Input: part model. Units: mm. Frame: model coordinates. A direction names the side the tool comes from. Coordinates: 2 decimals unless noted, no trailing zeros. Write each loop counter-clockwise with the first axis right and the second up, starting at its lowest first coordinate (ties: lowest second). Pieces come first, ordered by that corner, then holes. Notation, with made-up numbers: M 22.25,52 L 55.25,52 A37 cw 55.25,90 Z; hole C 69,25 d11. An arc over 180 degrees is marked long. Use one line per item in the form item = value.
from build123d import *

# Parameters (mm, degrees)
SKETCH_1_W                  = 78
SKETCH_1_H                  = 119.63
SKETCH_1_R                  = 22.5
EXTRUDE_1_DEPTH             = 8
HOLE_WIZARD_M5_1_AT_2_COUNT = 2
HOLE_WIZARD_M5_1_AT_2_PITCH = 58
SKETCH_4_W                  = 78
SKETCH_4_H                  = 23.52391086
EXTRUDE_2_DEPTH             = 8
SKETCH_5_W                  = 78
SKETCH_5_H                  = 8.43
EXTRUDE_3_DEPTH             = 10
SKETCH_6_W                  = 78
SKETCH_6_H                  = 18
CUT_EXTRUDE_1_DEPTH         = 0.43
SKETCH_7_R                  = 2.75
CUT_EXTRUDE_2_DEPTH         = 9
HOLE_WIZARD_M5_2_AT_2_COUNT = 2
HOLE_WIZARD_M5_2_AT_2_PITCH = 90


with BuildPart() as part:
    # 草图1 → 凸台-拉伸1 (new body)
    with BuildSketch(Plane.XY):
        with Locations((-39, 59.815)):
            Rectangle(SKETCH_1_W, SKETCH_1_H)
        with Locations((-39, 59.815)):
            Circle(SKETCH_1_R, mode=Mode.SUBTRACT)
    extrude(amount=EXTRUDE_1_DEPTH)

    # 草图3 → M5 螺纹孔1 (revolve, cut)
    with BuildSketch(Plane(origin=(-68, 119.63, 4), x_dir=(0, 0, 1), z_dir=(1, 0, 0))):
        Polygon((0, 0), (0, 13.6618073), (2.1, 12.4), (2.1, 0), align=None)
    hole_wizard_m5_1 = revolve(axis=Axis((-68, 125.98, 4), (0, -1, 0)), mode=Mode.SUBTRACT)

    # M5 螺纹孔1 at 2: M5 螺纹孔1 ×2
    with Locations(*[(i * HOLE_WIZARD_M5_1_AT_2_PITCH, 0, 0) for i in range(1, HOLE_WIZARD_M5_1_AT_2_COUNT)]):
        add(hole_wizard_m5_1, mode=Mode.SUBTRACT)

    # 镜向1: M5 螺纹孔1 across plane
    add(hole_wizard_m5_1.mirror(Plane.ZX.offset(59.815)), mode=Mode.SUBTRACT)

    # 镜向1 copy 1 sketch → 镜向1 copy 1 (revolve, cut)
    with BuildSketch(Plane(origin=(-10, 0, 4), x_dir=(0, 0, 1), z_dir=(1, 0, 0))):
        Polygon((0, 0), (0, -13.6618073), (2.1, -12.4), (2.1, 0), align=None)
    revolve(axis=Axis((-10, -6.35, 4), (0, -1, 0)), mode=Mode.SUBTRACT)

    # 草图4 → 凸台-拉伸2 (add)
    with BuildSketch(Plane.XY.offset(8)):
        with Locations((-39, 107.86804457)):
            Rectangle(SKETCH_4_W, SKETCH_4_H)
    extrude(amount=-EXTRUDE_2_DEPTH)

    # 草图5 → 凸台-拉伸3 (add)
    with BuildSketch(Plane(origin=(0, 0, 0), x_dir=(-1, 0, 0), z_dir=(0, 0, -1))):
        with Locations((39, 115.415)):
            Rectangle(SKETCH_5_W, SKETCH_5_H)
    extrude(amount=EXTRUDE_3_DEPTH)

    # 草图6 → 切除-拉伸1 (cut)
    with BuildSketch(Plane(origin=(0, 119.63, 0), x_dir=(1, 0, 0), z_dir=(0, 1, 0))):
        with Locations((-39, 1)):
            Rectangle(SKETCH_6_W, SKETCH_6_H)
    extrude(amount=-CUT_EXTRUDE_1_DEPTH, mode=Mode.SUBTRACT)

    # 草图7 → 切除-拉伸2 (cut, through all)
    with BuildSketch(Plane.XZ.offset(-111.2)):
        with Locations((-59, -5)):
            Circle(SKETCH_7_R)
        with Locations((-19, -5)):
            Circle(SKETCH_7_R)
    extrude(amount=-CUT_EXTRUDE_2_DEPTH, mode=Mode.SUBTRACT)

    # 草图9 → M5 螺纹孔2 (revolve, cut)
    with BuildSketch(Plane(origin=(-78, 7, 4), x_dir=(0, 0, 1), z_dir=(0, 1, 0))):
        Polygon((0, 0), (0, 7.2618073), (2.1, 6), (2.1, 0), align=None)
    hole_wizard_m5_2 = revolve(axis=Axis((-84.35, 7, 4), (1, 0, 0)), mode=Mode.SUBTRACT)

    # M5 螺纹孔2 at 2: M5 螺纹孔2 ×2
    with Locations(*[(0, 0, -i * HOLE_WIZARD_M5_2_AT_2_PITCH) for i in range(1, HOLE_WIZARD_M5_2_AT_2_COUNT)]):
        add(hole_wizard_m5_2, mode=Mode.SUBTRACT)

    # 镜向2: M5 螺纹孔2 across plane
    add(hole_wizard_m5_2.mirror(Plane(origin=(-39, 0, 0), x_dir=(0, 0, 1), z_dir=(1, 0, 0))), mode=Mode.SUBTRACT)

    # 镜向2 copy 1 sketch → 镜向2 copy 1 (revolve, cut)
    with BuildSketch(Plane(origin=(0, 7, -86), x_dir=(0, 0, 1), z_dir=(0, 1, 0))):
        Polygon((0, 0), (0, -7.2618073), (2.1, -6), (2.1, 0), align=None)
    revolve(axis=Axis((6.35, 7, -86), (1, 0, 0)), mode=Mode.SUBTRACT)


solid = part.part
(1) Line query: probe 1 along X at (y, z) = (3.5, 4); probe 2 along Z at (x, y) = (-19, 113.5); probe 3 along X at (y, z) = (6, 4). Output: solid intervals per line, ascending.
Computed:
probe_1 = -78 to -70.1, -65.9 to -12.1, -7.9 to 0
probe_2 = -10 to -7.75, -2.25 to 8
probe_3 = -71.34 to -70.1, -65.9 to -12.1, -7.9 to -6.66
(2) Set-up query: faces 5 (the cylindrical face through (-75.04, 5.23, 5.13)), 6 (the cylindrical face through (-11.77, 6.11, 5.13)), 7 (the flat face through (-38, 115, -10)), 8 (the flat face through (-38, 111.2, -5)). Return all of +Z, -Z, +X, -X, +Y, -Y with unobstructed straight access to the full face (end or side cutting, diameter ignored); none if empty.
Computed:
face_5 = -X
face_6 = -Y
face_7 = -Z, +X, -X, +Y, -Y
face_8 = -Z, +X, -X, -Y
(3) First-contact query: pin 1 Ø5 at (x, z) = (-19, -5) entering from +Y; pin 2 Ø10 at (x, y) = (-66, 98.5) entering from -Z; pin 3 Ø5 at (x, z) = (-56.5, -4.5) entering from -Y. Flat tips, straight axial feed; report the tip coordinate or a pass-through.
Computed:
pin_1 = through
pin_2 = 0
pin_3 = 111.2
(4) Section query B-B on x = -19. Return the cut outline in (y, z), plus the area to 3 significant figures.
Computed:
outline = M 0,0 L 49.51,0 L 49.51,8 L 0,8 Z; M 70.12,0 L 111.2,0 L 111.2,-2.25 L 119.2,-2.25 L 119.2,8 L 70.12,8 Z; M 111.2,-10 L 119.2,-10 L 119.2,-7.75 L 111.2,-7.75 Z
area = 825 mm^2
(5) Section query A-A on x = -39. Return the cut outline in (y, z) (3 decimals), plus the area to 3 significant figures.
Computed:
outline = M 0,0 L 37.315,0 L 37.315,8 L 0,8 Z; M 82.315,0 L 111.2,0 L 111.2,-10 L 119.2,-10 L 119.2,8 L 82.315,8 Z
area = 674 mm^2
(6) Section query D-D on y = 99. Return the cut outline in (x, z).
Computed:
outline = M -78,0 L 0,0 L 0,8 L -78,8 Z
(7) Section query C-C on y = 40.5. Return the cut outline in (x, z).
Computed:
outline = M -78,0 L -50.54,0 L -50.54,8 L -78,8 Z; M -27.46,0 L 0,0 L 0,8 L -27.46,8 Z
(8) Pull-direction query (Y, two-part tool) for faces 1 (the cylindrical face through (-2.96, 5.23, 5.13)), 2 (the cylindrical face through (-61.747, 115.144, -4.879)), 3 (the cylindrical face through (-28.618, 39.854, 3.944)), 4 (the flat face through (-40, 0, 4)); classes: pulls with the +Y half, pulls with the -Y half, needs draft (parallel to the pull), parting line crosses it, or undercut.
Computed:
face_1 = undercut
face_2 = needs draft
face_3 = undercut
face_4 = pulls with the -Y half
